```python
from build123d import *

# Parameters (mm, degrees)
SKETCH1_W                                       = 15.875
SKETCH1_H                                       = 25.4
BOSS_EXTRUDE1_DEPTH                             = 12.7
SKETCH2_R                                       = 8.255
SKETCH2_W                                       = 3.175
SKETCH2_H                                       = 12.7
CUT_EXTRUDE1_DEPTH                              = 24.970724332
CBORE_FOR_10_SOCKET_HEAD_CAP_SCREW1_D           = 5.1054
CBORE_FOR_10_SOCKET_HEAD_CAP_SCREW1_CBORE_D     = 9.525
CBORE_FOR_10_SOCKET_HEAD_CAP_SCREW1_CBORE_DEPTH = 4.826
FILLET2_R                                       = 2.54
CUT_EXTRUDE2_DEPTH                              = 6.207125


with BuildPart() as part:
    # Sketch1 → Boss-Extrude1 (new, symmetric)
    with BuildSketch(Plane.XY):
        Rectangle(SKETCH1_W, SKETCH1_H)
    extrude(amount=BOSS_EXTRUDE1_DEPTH, both=True)

    # Sketch2 → Cut-Extrude1 (cut, through all)
    with BuildSketch(Plane(origin=(7.9375, 0, 0), x_dir=(0, 0, -1), z_dir=(1, 0, 0))):
        with Locations((0, -12.7)):
            Circle(SKETCH2_R)
        with Locations((0, 6.35)):
            Rectangle(SKETCH2_W, SKETCH2_H)
    extrude(amount=-CUT_EXTRUDE1_DEPTH, mode=Mode.SUBTRACT)

    # CBORE for #10 Socket Head Cap Screw1 (through all)
    with Locations(Plane.XY.offset(12.7)):
        with Locations((0, 6.35)):
            CounterBoreHole(CBORE_FOR_10_SOCKET_HEAD_CAP_SCREW1_D / 2, CBORE_FOR_10_SOCKET_HEAD_CAP_SCREW1_CBORE_D / 2, CBORE_FOR_10_SOCKET_HEAD_CAP_SCREW1_CBORE_DEPTH)

    # Fillet2
    # the kernel refuses this fillet: 2.54 mm, written as the material it takes off along each edge
    with BuildSketch(Plane(origin=(13.529804731, -12.7, -8.255), x_dir=(0, 0, -1), z_dir=(-1, 0, 0))) as fillet2_piece_1:
        with BuildLine():
            CenterArc((2.236921893, -2.54), FILLET2_R, 90, 76.391039369)
            ThreePointArc((-0.231765612, -1.942352941), (-0.058146187, -0.978065725), (0, 0))
            Line((0, 0), (2.236921893, 0))
        make_face()
    extrude(amount=27.059609463, mode=Mode.SUBTRACT)
    with BuildSketch(Plane(origin=(-13.529804731, -12.7, 8.255), x_dir=(0, 0.9929562463238144, -0.11848161412860811), z_dir=(1, 0, 0))) as fillet2_piece_2:
        with BuildLine():
            CenterArc((2.257074749, 2.522108866), FILLET2_R, 186.804480315, 76.391039369)
            Line((-0.265034117, 2.221165566), (0, 0))
            ThreePointArc((0, 0), (0.978065725, 0.058146187), (1.956131449, 0))
        make_face()
    extrude(amount=27.059609463, mode=Mode.SUBTRACT)
    with BuildSketch(Plane(origin=(14.2875, 12.7, 12.7), x_dir=(0, 0, -1), z_dir=(-1, 0, 0)), Plane(origin=(14.2875, 12.7, -12.7), x_dir=(0, -1, 0), z_dir=(-1, 0, 0)), Plane(origin=(14.2875, 12.7, -1.5875), x_dir=(0, 0, -1), z_dir=(-1, 0, 0)), Plane(origin=(14.2875, 12.7, 1.5875), x_dir=(0, -1, 0), z_dir=(-1, 0, 0))) as fillet2_piece_3:
        with BuildLine():
            CenterArc((FILLET2_R, FILLET2_R), FILLET2_R, 180, 90)
            Line((0, FILLET2_R), (0, 0))
            Line((0, 0), (FILLET2_R, 0))
        make_face()
    extrude(amount=28.575, mode=Mode.SUBTRACT)
    with BuildSketch(Plane(origin=(-14.2875, -12.7, 12.7), x_dir=(0, 1, 0), z_dir=(1, 0, 0)), Plane(origin=(-14.2875, -12.7, -12.7), x_dir=(0, 0, 1), z_dir=(1, 0, 0))) as fillet2_piece_4:
        with BuildLine():
            CenterArc((FILLET2_R, -FILLET2_R), FILLET2_R, 90, 90)
            Line((0, -FILLET2_R), (0, 0))
            Line((0, 0), (FILLET2_R, 0))
        make_face()
    extrude(amount=28.575, mode=Mode.SUBTRACT)

    # Sketch5 → Cut-Extrude2 (cut)
    with BuildSketch(Plane(origin=(0, 0, -12.7), x_dir=(-1, 0, 0), z_dir=(0, 0, -1))):
        Polygon((5.645908282, 6.35), (2.822954141, 11.2395), (-2.822954141, 11.2395), (-5.645908282, 6.35), (-2.822954141, 1.4605), (2.822954141, 1.4605), align=None)
    extrude(amount=-CUT_EXTRUDE2_DEPTH, mode=Mode.SUBTRACT)


solid = part.part
```
Verification items for the finished model (mm, model axes). A direction names the side the tool comes from. Round coordinates to 2 decimals unless told otherwise and drop trailing zeros. Order: outer loops, then holes, each group sorted by start corner. A loop starts at its lowest first (then second) coordinate and runs counter-clockwise, first axis right, second up. Notation, with made-up numbers: (34.25, 77) - (79.25, 77) arc R27 cw to (79.25, 108) - close; hole circle Ø3 at (-7.5, -21.5). An arc over 180 degrees is marked (long way). Use CSV: the item, a comma, the result in double quotes.
(1) Access from +Z, -Z, +X, -X, +Y, -Y to the whole of each face (thin tool, end or side, straight path). Record for faces 1 (the face through (-0.111, -12.118, 8.874)), 2 (the face through (1, 9, -6.493)), 3 (the face through (0, -2, -12.7)), 4 (the face through (0.111, 11.976, -11.936)), 5 (the face through (2, 4, -1.588)).
Entries:
face 1,"+X, -X, -Y"
face 2,"-Z"
face 3,"-Z, +X, -X, +Y, -Y"
face 4,"-Z, +X, -X, +Y"
face 5,"+X, -X, +Y"
(2) Section check D-D on z = -6. Record the boundary of the cut face in (x, y), and give its area (3 significant figures).
Entries:
outline,"(-7.94, -7.03) - (7.94, -7.03) - (7.94, 12.7) - (-7.94, 12.7) - close; hole circle Ø5.11 at (0, 6.35)"
area,"293 mm^2"
(3) Section check B-B on z = 7. Record the boundary of the cut face in (x, y), and give its area (3 significant figures).
Entries:
outline,"(-7.94, -8.32) - (7.94, -8.32) - (7.94, 12.7) - (-7.94, 12.7) - close; hole circle Ø5.11 at (0, 6.35)"
area,"313 mm^2"
(4) Thickness scan on probe 1 along X at (y, z) = (6.35, 10.4); probe 2 along Z at (x, y) = (2, 3.5); probe 3 along Z at (x, y) = (-4.75, 9). Record the ranges inside material, lowest first. Write a range as from..to.
Entries:
probe 1,"-7.94..-4.76, 4.76..7.94"
probe 2,"-6.49..-1.59, 1.59..7.87"
probe 3,"-12.7..-1.59, 1.59..12.7"
(5) Section check A-A on x = 0. State how many separate pieces and enclosed holes the cut face has, and give its area (3 significant figures).
Entries:
separate pieces,"3"
enclosed holes,"0"
area,"324 mm^2"
(6) Mould release check, pull along X, two halves, no side actions. Record for faces 6 (the face through (-4.254, 8.761, -9.64)), 7 (the face through (0, -2, 12.7)), 8 (the face through (0, 1.46, -10)): released by +X, released by -X, zero draft, split by the parting line, or undercut.
Entries:
face 6,"undercut"
face 7,"zero draft"
face 8,"undercut"
(7) Section check C-C on x = -6. Record the boundary of the cut face in (y, z) (1 decimal).
Entries:
outline,"(-12.7, -10.3) arc R2.5 ccw to (-10.2, -12.7) - (10.2, -12.7) arc R2.5 ccw to (12.7, -10.2) - (12.7, -4.1) arc R2.5 ccw to (10.2, -1.6) - (0, -1.6) - (0, 1.6) - (10.2, 1.6) arc R2.5 ccw to (12.7, 4.1) - (12.7, 10.2) arc R2.5 ccw to (10.2, 12.7) - (-10.2, 12.7) arc R2.5 ccw to (-12.7, 10.3) arc R2.5 ccw to (-10.8, 8) arc R8.3 cw to (-10.8, -8) arc R2.5 ccw to start"
(8) Gauge pin test, flat ends, axial feed: pin 1 Ø1 at (x, z) = (3, 0.5) entering from +Y; pin 2 Ø5 at (x, z) = (6.5, -1) entering from -Y; pin 3 Ø7.5 at (x, y) = (0, 6.35) entering from +Z. Record the tip position at first contact, or that the pin passes through.
Entries:
pin 1,"y = 0"
pin 2,"y = -5.22"
pin 3,"z = 7.87"
